Geometry check sheet. Reference: the model listing, model coordinates, mm. A direction names the side the tool comes from. Round coordinates to 2 decimals unless told otherwise and drop trailing zeros. Write each loop counter-clockwise with the first axis right and the second up, starting at its lowest first coordinate (ties: lowest second). Pieces come first, ordered by that corner, then holes. Notation, with made-up numbers: M 10,-18 L 68,-18 A13 cw 68,3 Z; hole C 10.5,-8.5 d4. An arc over 180 degrees is marked long. Put each result on its own line as item: value. Start each with the question number.
(1) Mould release check, pull along Y, two halves, no side actions. Record for faces 3 (the flat face through (2.7, 5, -78.6)), 4 (the flat face through (2, 0, -49)), 5 (the flat face through (10, 25, -39)): pulls with the +Y half, pulls with the -Y half, needs draft (parallel to the pull), parting line crosses it, or undercut.
(2) Section check A-A on z = -50. Record the cut outline in (x, y).
(3) Tool access check on faces 1 (the cylindrical face through (5.1, 7, -12.1)), 2 (the flat face through (0, 25.4, -60.4)). Record the directions out of +Z, -Z, +X, -X, +Y, -Y that give a thin tool (end or side, any length) a straight path to the whole face; none if there is none.
(4) Section check B-B on y = 28.5. Record the cut outline in (x, z).
(5) Section check C-C on x = 5. Count the separate pieces of the cut face and the enclosed holes in it, then the cut area to 3 significant figures.
(6) Section check D-D on z = -79. Record the cut outline in (x, y), then the cut area to 3 significant figures.
(7) Gauge pin test, flat ends, axial feed: pin 1 (3 mm diameter, centred on x = 7, z = -79.5, fed in from -Y); pin 2 (1.8 mm diameter, centred on x = 5.5, z = -19.5, fed in from -Y); pin 3 (2 mm diameter, centred on x = 8.5, y = 22, fed in from -Z). Record the tip position at first contact, or that the pin passes through.
(8) Material ranges on probe 1 along Z at (x, y) = (3.25, 23); probe 2 along Y at (x, z) = (2.5, -83); probe 3 along X at (y, z) = (47.05, -80), recorded low to high.
from build123d import *

# Parameters (mm, degrees)
ESQUISSE1_W             = 100
ESQUISSE1_H             = 50
ESQUISSE1_W_2           = 80
ESQUISSE1_H_2           = 40
ESQUISSE1_W_3           = 10
BOSS_EXTRU_1_DEPTH      = 10
ESQUISSE2_R             = 2.4
ENL_V_MAT_EXTRU_1_DEPTH = 113.249721603
CONG_1_R                = 7
CONG_2_R                = 3


with BuildPart() as part:
    # Esquisse1 → Boss.-Extru.1 (new body)
    # profile 1 of 3: a face of its own
    with BuildSketch(Plane(origin=(0, 0, 0), x_dir=(0, 0, -1), z_dir=(1, 0, 0))):
        with Locations((50, 25)):
            Rectangle(ESQUISSE1_W, ESQUISSE1_H)
        with Locations((50, 25)):
            Rectangle(ESQUISSE1_W_2, ESQUISSE1_H_2, mode=Mode.SUBTRACT)
    # profile 2 of 3: a face of its own
    with BuildSketch(Plane(origin=(0, 0, 0), x_dir=(0, 0, -1), z_dir=(1, 0, 0))):
        with Locations((65, 25)):
            Rectangle(ESQUISSE1_W_3, ESQUISSE1_H_2)
    # profile 3 of 3: a face of its own
    with BuildSketch(Plane(origin=(0, 0, 0), x_dir=(0, 0, -1), z_dir=(1, 0, 0))):
        with Locations((35, 25)):
            Rectangle(ESQUISSE1_W_3, ESQUISSE1_H_2)
    extrude(amount=BOSS_EXTRU_1_DEPTH)

    # Esquisse2 → Enlèv. mat.-Extru.1 (cut, through all)
    with BuildSketch(Plane.XZ):
        with Locations(Location((5, -20, 0), (0, 0, 270))):
            Circle(ESQUISSE2_R)
        with Locations(Location((5, -50, 0), (0, 0, 270))):
            Circle(ESQUISSE2_R)
        with Locations(Location((5, -80, 0), (0, 0, 270))):
            Circle(ESQUISSE2_R)
    extrude(amount=-ENL_V_MAT_EXTRU_1_DEPTH, mode=Mode.SUBTRACT)

    # Congé1
    cong_1_edges = [part.edges().sort_by_distance(p)[0] for p in [
        (5, 5, -30),
        (5, 45, -30),
        (5, 45, -10),
        (5, 5, -10),
        (5, 5, -90),
        (5, 45, -90),
        (5, 45, -70),
        (5, 5, -70),
        (5, 5, -60),
        (5, 45, -60),
        (5, 45, -40),
        (5, 5, -40),
    ]]
    fillet(cong_1_edges, radius=CONG_1_R)

    # Congé2
    cong_2_edges = [part.edges().sort_by_distance(p)[0] for p in [
        (10, 25, 0),
        (10, 25, -100),
    ]]
    fillet(cong_2_edges, radius=CONG_2_R)


solid = part.part
Answers follow:
1. face 3: undercut
1. face 4: pulls with the -Y half
1. face 5: needs draft
2. outline: M 0,0 L 2.6,0 L 2.6,5 L 0,5 Z; M 0,45 L 2.6,45 L 2.6,50 L 0,50 Z; M 7.4,0 L 10,0 L 10,5 L 7.4,5 Z; M 7.4,45 L 10,45 L 10,50 L 7.4,50 Z
3. face 1: +X, -X
3. face 2: +Z, -Z, -X, +Y, -Y
4. outline: M 0,-100 L 7,-100 A3 ccw 10,-97 L 10,-90 L 0,-90 Z; M 0,-70 L 10,-70 L 10,-60 L 0,-60 Z; M 0,-40 L 10,-40 L 10,-30 L 0,-30 Z; M 0,-10 L 10,-10 L 10,-3 A3 ccw 7,0 L 0,0 Z
5. separate pieces: 4
5. enclosed holes: 0
5. area: 2,580 mm^2
6. outline: M 0,0 L 2.82,0 L 2.82,5 L 0,5 Z; M 0,45 L 2.82,45 L 2.82,50 L 0,50 Z; M 7.18,0 L 10,0 L 10,5 L 7.18,5 Z; M 7.18,45 L 10,45 L 10,50 L 7.18,50 Z
6. area: 56.4 mm^2
7. pin 1: stops at y = 0
7. pin 2: passes through
7. pin 3: stops at z = -99.96
8. probe 1: z = -100 to -90, -70 to -60, -40 to -30, -10 to 0
8. probe 2: y = 0 to 5, 45 to 50
8. probe 3: x = 0 to 2.6, 7.4 to 10
